Could you check a few things on this model? Use its own coordinates, in mm. A direction names the side the tool comes from. Give positions to 0.01 mm unless a question says otherwise; leave off trailing zeros. Order: outer loops, then holes, each group sorted by start corner. A loop starts at its lowest first (then second) coordinate and runs counter-clockwise, first axis right, second up. Notation, with made-up numbers: (-37, 45) -> (1, 45) arc R33 cw to (1, 82) -> close; hole circle Ø4 at (19.25, 13.5). An arc over 180 degrees is marked (long way). Answer as CSV lines item,"result". Start each with the question number.
(1) We'd pull the mould along Y, two halves only. Please class faces 1 (the face through (13, -6, -2)), 2 (the face through (1.48, -3.47, 15.62)), 3 (the face through (1.48, 13.4, 0.33)): released by +Y, released by -Y, zero draft, split by the parting line, or undercut.
(2) Will these pins go through, and if not, where does the flat tip stop? pin 1 Ø5 at (y, z) = (11.938, 0) entering from +X; pin 2 Ø6 at (x, z) = (8.5, 0) entering from +Y; pin 3 Ø1.5 at (x, y) = (9, -7.5) entering from -Z.
(3) On a 3-axis mill with a long thin cutter (end or side, diameter ignored), from which of +Z, -Z, +X, -X, +Y, -Y can I reach the whole of each face in a straight line? I mean faces 4 (the face through (1.48, -0.07, -10.44)), 5 (the face through (3, 7, -7)). Say none if no direction works.
(4) I need wall thicknesses on L1, parallel to Y at x = 4.75, z = 0; L2, parallel to Y at x = 1, z = -0.5; L3, parallel to X at y = -3.5, z = -13. Which ranges of each line are inside material? Lowest first, please.
(5) I want a section at D-D (y = -4). Please give me the cut outline in (x, z).
(6) I want a section at A-A (y = 0). Please give me the cut outline in (x, z), plus the area to 3 significant figures.
(7) I want a section at C-C (z = 12). Please give me the cut outline in (x, y), plus the area to 3 significant figures.
Autodesk Inventor part; units mm, degrees
ref_plane "YZ Plane" through (0, 0, 0) normal (1, 0, 0) x (0, 1, 0)
ref_plane "XZ Plane" through (0, 0, 0) normal (0, 1, 0) x (-1, 0, 0)
ref_plane "XY Plane" through (0, 0, 0) normal (0, 0, 1) x (1, 0, 0)
sketch "Sketch1" plane through (0, 0, 0) normal (1, 0, 0) x (0, 1, 0)
  circle A0 centre (0, 0) radius 16
  dimension "d0" = 32
extrude "Extrusion1" add sketch "Sketch1" along normal blind 3
sketch "Sketch2" plane through (3, 0, 0) normal (1, 0, 0) x (0, 0, -1)
  circle A0 centre (0, 0) radius 9
  dimension "d3" = 18
extrude "Extrusion2" add sketch "Sketch2" along normal blind 10
sketch "Sketch3" plane through (13, 0, 0) normal (1, 0, 0) x (0, 0, -1)
  circle A0 centre (0, 0) radius 6
  dimension "d6" = 12
extrude "Extrusion3" cut sketch "Sketch3" against normal through all
sketch "Sketch4" plane through (3, 0, 0) normal (1, 0, 0) x (0, 0, -1)
  circle A0 centre (0, 0) radius 9
  circle A1 centre (0, 0) radius 16
  point P0 (0, 11.938)
  point P1 (-11.938, 0)
  point P2 (0, -11.938)
  point P3 (11.938, 0)
  dimension "d9" = 11.938
  dimension "d10" = 32
  dimension "d11" = 18
  dimension "d14" = 360
hole "Hole1" at (3, 11.938, 0) at (3, 0, 11.938) at (3, -11.938, 0) at (3, 0, -11.938) direction (-1, 0, 0) diameter 3 end through all
properties part number "Flange"
Final values:
1,face 1,"zero draft"
1,face 2,"split by the parting line"
1,face 3,"undercut"
2,pin 1,"x = 3"
2,pin 2,"y = 9"
2,pin 3,"z = -5.95"
3,face 4,"+X, -X"
3,face 5,"+X"
4,L1,"-9 to -6, 6 to 9"
4,L2,"-15.99 to -13.35, -10.52 to -5.98, 5.98 to 10.52, 13.35 to 15.99"
4,L3,"0 to 3"
5,outline,"(0, -15.49) -> (3, -15.49) -> (3, -8.06) -> (13, -8.06) -> (13, -4.47) -> (0, -4.47) -> close; (0, 4.47) -> (13, 4.47) -> (13, 8.06) -> (3, 8.06) -> (3, 15.49) -> (0, 15.49) -> close"
6,outline,"(0, -16) -> (3, -16) -> (3, -13.44) -> (0, -13.44) -> close; (0, -10.44) -> (3, -10.44) -> (3, -9) -> (13, -9) -> (13, -6) -> (0, -6) -> close; (0, 6) -> (13, 6) -> (13, 9) -> (3, 9) -> (3, 10.44) -> (0, 10.44) -> close; (0, 13.44) -> (3, 13.44) -> (3, 16) -> (0, 16) -> close"
6,area,"102 mm²"
7,outline,"(0, -10.58) -> (3, -10.58) -> (3, -1.5) -> (0, -1.5) -> close; (0, 1.5) -> (3, 1.5) -> (3, 10.58) -> (0, 10.58) -> close"
7,area,"54.5 mm²"
